Design review of the part built by this model. Coordinates are the model's own, in mm. Face numbers are marked on the shaded views. Coordinates: 2 decimals unless noted, no trailing zeros. Write each loop counter-clockwise with the first axis right and the second up, starting at its lowest first coordinate (ties: lowest second). Pieces come first, ordered by that corner, then holes. Notation, with made-up numbers: M 73,-18.75 L 90,-18.75 A21 cw 90,18.25 Z; hole C 25.5,51.5 d4. An arc over 180 degrees is marked long. One line per question, with ' | ' between items.
from build123d import *

# Parameters (mm, degrees)
SKETCH1_R                = 5.5
BOSS_EXTRUDE1_DEPTH      = 15
SKETCH2_R                = 2.5
BOSS_EXTRUDE2_DEPTH      = 64
SKETCH3_R                = 2.5
CUT_EXTRUDE1_DEPTH       = 8
BOSS_EXTRUDE3_DEPTH      = 2.5
BOSS_EXTRUDE3_DEPTH_BACK = 7.5
SKETCH4_R                = 1


with BuildPart() as part:
    # Sketch1 → Boss-Extrude1 (new body)
    with BuildSketch(Plane(origin=(0, 0, 0), x_dir=(0, 0, -1), z_dir=(1, 0, 0))):
        Circle(SKETCH1_R)
    extrude(amount=BOSS_EXTRUDE1_DEPTH)

    # Sketch2 → Boss-Extrude2 (add)
    with BuildSketch(Plane(origin=(15, 0, 0), x_dir=(0, 0, -1), z_dir=(1, 0, 0))):
        Circle(SKETCH2_R)
    extrude(amount=BOSS_EXTRUDE2_DEPTH)

    # Sketch3 → Cut-Extrude1 (cut)
    with BuildSketch(Plane.ZY):
        with Locations(Location((0, 0, 0), (0, 0, 180))):
            Circle(SKETCH3_R)
    extrude(amount=-CUT_EXTRUDE1_DEPTH, mode=Mode.SUBTRACT)

    # Sketch4 → Boss-Extrude3 (add, two sides: drawn at the far end of the back side and taken through both)
    with BuildSketch(Plane.XY.offset(2.5).offset(-BOSS_EXTRUDE3_DEPTH_BACK)):
        with Locations((76.405258654, 0)):
            Circle(SKETCH4_R)
    extrude(amount=BOSS_EXTRUDE3_DEPTH + BOSS_EXTRUDE3_DEPTH_BACK)


solid = part.part
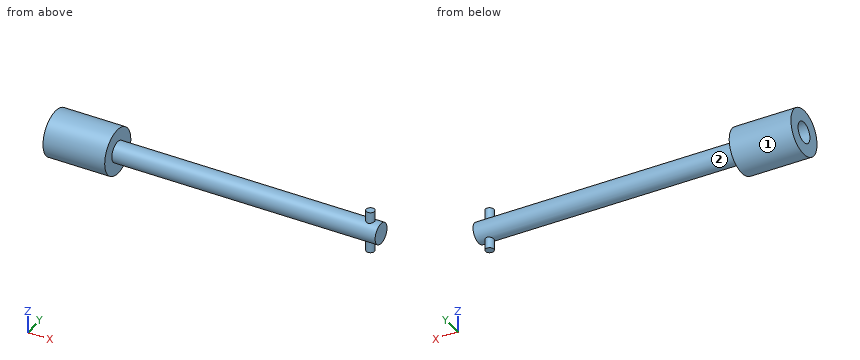
1. Take a section at C-C (x = 11). Write out the cut boundary in (y, z), then the cut area to 3 significant figures.
Answer sheet:
outline: C 0,0 d11 | area: 95.0 mm^2
2. Take a section at A-A (y = 0). Write out the cut boundary in (x, z), then the cut area to 3 significant figures.
Answer sheet:
outline: M 0,-5.5 L 15,-5.5 L 15,-2.5 L 75.41,-2.5 L 75.41,-5 L 77.41,-5 L 77.41,-2.5 L 79,-2.5 L 79,2.5 L 77.41,2.5 L 77.41,5 L 75.41,5 L 75.41,2.5 L 15,2.5 L 15,5.5 L 0,5.5 L 0,2.5 L 8,2.5 L 8,-2.5 L 0,-2.5 Z | area: 455 mm^2
3. Take a section at D-D (x = 57). Write out the cut boundary in (y, z), then the cut area to 3 significant figures.
Answer sheet:
outline: C 0,0 d5 | area: 19.6 mm^2
4. To check wall thickness, follow line 1 along Y through (x, z) = (3, 0); line 2 along X through (y, z) = (-1.25, -4.25); line 3 along X through (y, z) = (-0.75, 0). State the ranges of each line that lie inside material, in increasing order. Write a range as [from, to].
Answer sheet:
line 1: [-5.5, -2.5], [2.5, 5.5] | line 2: [0, 15] | line 3: [8, 79]
5. Insertion check: pin 1 Ø4 at (x, y) = (50, 3.5) entering from -Z; pin 2 Ø1.5 at (x, z) = (57, 1.5) entering from +Y; pin 3 Ø5 at (x, z) = (59, 0) entering from -Y. Each pin has a flat end and moves straight along its axis. Give the tip position at first contact, or say it passes through.
Answer sheet:
pin 1: z = -2 | pin 2: y = 2.38 | pin 3: y = -2.5
6. Take a section at B-B (z = 0). Write out the cut boundary in (x, y), then the cut area to 3 significant figures.
Answer sheet:
outline: M 0,-5.5 L 15,-5.5 L 15,-2.5 L 79,-2.5 L 79,2.5 L 15,2.5 L 15,5.5 L 0,5.5 L 0,2.5 L 8,2.5 L 8,-2.5 L 0,-2.5 Z | area: 445 mm^2
7. Draft analysis for pull direction X (two halves, no side actions). For the marked faces 1 and 2, state which applies: pulls with the +X half, pulls with the -X half, needs draft (parallel to the pull), parting line crosses it, or undercut.
Answer sheet:
face 1: needs draft | face 2: undercut
